Could you check a few things on this model? Use its own coordinates, in mm. Face numbers are marked on the shaded views. A direction names the side the tool comes from. Give positions to 0.01 mm unless a question says otherwise; leave off trailing zeros. Order: outer loops, then holes, each group sorted by start corner. A loop starts at its lowest first (then second) coordinate and runs counter-clockwise, first axis right, second up. Notation, with made-up numbers: M 2,45 L 13,45 A12 ccw 13,59 Z; hole C 8,-25.5 d8. An arc over 180 degrees is marked long. Use a Markdown table: item, result. Add a question column.
Item 1: If I drill on L1, parallel to X at y = 19, z = -1.25; L2, parallel to Z at x = -1.75, y = 0; L3, parallel to Y at x = 0, z = -6 (3 decimals), over which ranges is the centre line in solid material (lowest first)? Write a range as from..to.
Item 2: Suppose I cut it at A-A on x = 0. Write out the boundary of the cut face in (y, z) (3 decimals), plus the area to 3 significant figures.
Item 3: Suppose I cut it at D-D on x = 2. Write out the boundary of the cut face in (y, z).
Item 4: Suppose I cut it at C-C on z = -2.5. Write out the boundary of the cut face in (x, y) (3 decimals).
Item 5: Suppose I cut it at B-B on y = 5.5. Write out the boundary of the cut face in (x, z) (3 decimals), plus the area to 3 significant figures.
Item 6: For the marked faces 1, 2 and 3, which set-ups out of +Z, -Z, +X, -X, +Y, -Y let a thin tool reach every point of the face, with its end or its side?
Item 7: I'm going to push flat-ended pins straight in: pin 1 Ø8 at (y, z) = (6, 6) entering from -X; pin 2 Ø1.5 at (y, z) = (10, 3) entering from -X. Where does each tip first touch, or does it pass through?
from build123d import *

# Parameters (mm, degrees)
SKETCH1_R           = 3.175
BOSS_EXTRUDE1_DEPTH = 31.75
SKETCH2_R           = 3.175
BOSS_EXTRUDE2_DEPTH = 12.7
DOME2_FACE_RADIUS   = 3.175
DOME2_HEIGHT        = 3.175


with BuildPart() as part:
    # Sketch1 → Boss-Extrude1 (new body)
    with BuildSketch(Plane(origin=(0, 0, 0), x_dir=(1, 0, 0), z_dir=(0, 1, 0))):
        Circle(SKETCH1_R)
    extrude(amount=BOSS_EXTRUDE1_DEPTH)

    # Sketch2 → Boss-Extrude2 (add, symmetric)
    with BuildSketch(Plane.XY):
        with Locations((0, 25.4)):
            Circle(SKETCH2_R)
    extrude(amount=BOSS_EXTRUDE2_DEPTH, both=True)

    # Dome2: a dome of height H over a round flat face of radius A is a cap of a sphere of radius (A * A + H * H) / (2 * H)
    dome2_r = (DOME2_FACE_RADIUS * DOME2_FACE_RADIUS + DOME2_HEIGHT * DOME2_HEIGHT) / (2 * DOME2_HEIGHT)
    dome2_base = Plane((0, 0, 0), z_dir=(0, -1, 0))
    with Locations(dome2_base.offset(DOME2_HEIGHT - dome2_r)):
        dome2_ball = Sphere(dome2_r, mode=Mode.PRIVATE)
    add(split(dome2_ball, bisect_by=dome2_base, keep=Keep.TOP, mode=Mode.PRIVATE))


solid = part.part
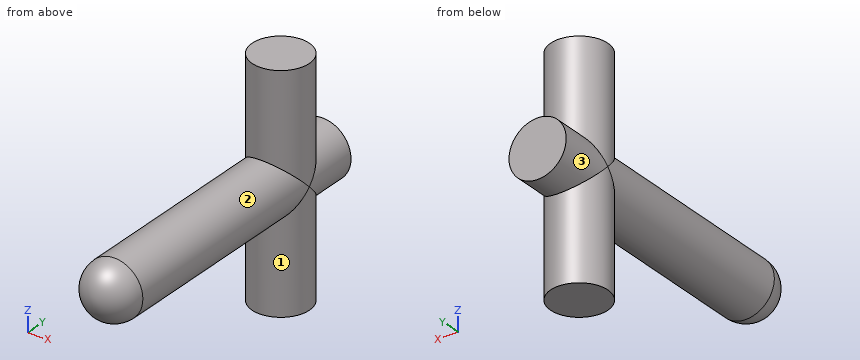
Findings below:
| question | item | result |
|---|---|---|
| 1 | L1 | x = -2.92..2.92 |
| 1 | L2 | z = -2.65..2.65 |
| 1 | L3 | y = 22.225..28.575 |
| 2 | outline | M 0,-3.175 L 22.225,-3.175 L 22.225,-12.7 L 28.575,-12.7 L 28.575,-3.175 L 31.75,-3.175 L 31.75,3.175 L 28.575,3.175 L 28.575,12.7 L 22.225,12.7 L 22.225,3.175 L 0,3.175 A3.175 ccw Z |
| 2 | area | 338 mm^2 |
| 3 | outline | M 0,-2.47 L 22.93,-2.47 L 22.93,-12.7 L 27.87,-12.7 L 27.87,-2.47 L 31.75,-2.47 L 31.75,2.47 L 27.87,2.47 L 27.87,12.7 L 22.93,12.7 L 22.93,2.47 L 0,2.47 A2.47 ccw Z |
| 4 | outline | M -1.957,0 A1.957 ccw 1.957,0 L 1.957,22.9 A3.175 ccw 1.957,27.9 L 1.957,31.75 L -1.957,31.75 L -1.957,27.9 A3.175 ccw -1.957,22.9 Z |
| 5 | outline | C 0,0 d6.35 |
| 5 | area | 31.7 mm^2 |
| 6 | face 1 | -Z |
| 6 | face 2 | -Y |
| 6 | face 3 | +Y |
| 7 | pin 1 | stops at x = -2.47 |
| 7 | pin 2 | stops at x = -2.24 |
